For this review, use the dimensioned drawing (mm, ordinates from the lowest corner) and the shaded views. Coordinates: 2 decimals unless noted, no trailing zeros. Order: outer loops, then holes, each group sorted by start corner. A loop starts at its lowest first (then second) coordinate and runs counter-clockwise, first axis right, second up. Notation, with made-up numbers: M -5,-30.75 L 49,-30.75 A10 ccw 49,-14.75 Z; hole C -12.75,63.25 d5. An arc over 180 degrees is marked long. Answer as CSV lines item,"result". Start each with the question number.
Q1. Wall thickness on L1, parallel to Y at x = 6.25, z = 7.75; L2, parallel to Z at x = 3.75, y = 1.25; L3, parallel to Z at x = 8.25, y = 6.5: over which ranges is each line inside the solid? List them lowest first. Write a range as [from, to].
Q2. The part is to be moulded in two halves that separate along X. For the marked faces 1, 2 and 3, say which applies: +X half, -X half, draft (parallel to the pull), parting line (faces both ways), or undercut.
Q3. Consider section D-D on y = 9.75. Write out the cut boundary in (x, z).
Q4. Consider section C-C on x = 8.8. Write out the cut boundary in (y, z).
Q5. For P1, Ø1.2, axis at x = 8.5, z = 6, coming from the -Y side; P2, Ø3, axis at x = 3.5, y = 7, coming from the +Z side; P3, Ø3, axis at x = 6.5, y = 1.5, coming from the +Z side; P4, Ø3, axis at y = 4.5, z = 3.5, coming from the -X side, all flat-tipped, find the tip position at first contact; note any pin that passes through.
Q6. Consider section A-A on z = 6.3. Write out the cut boundary in (x, y).
Q7. Consider section B-B on y = 2. Write out the cut boundary in (x, z), and give its area (3 significant figures).
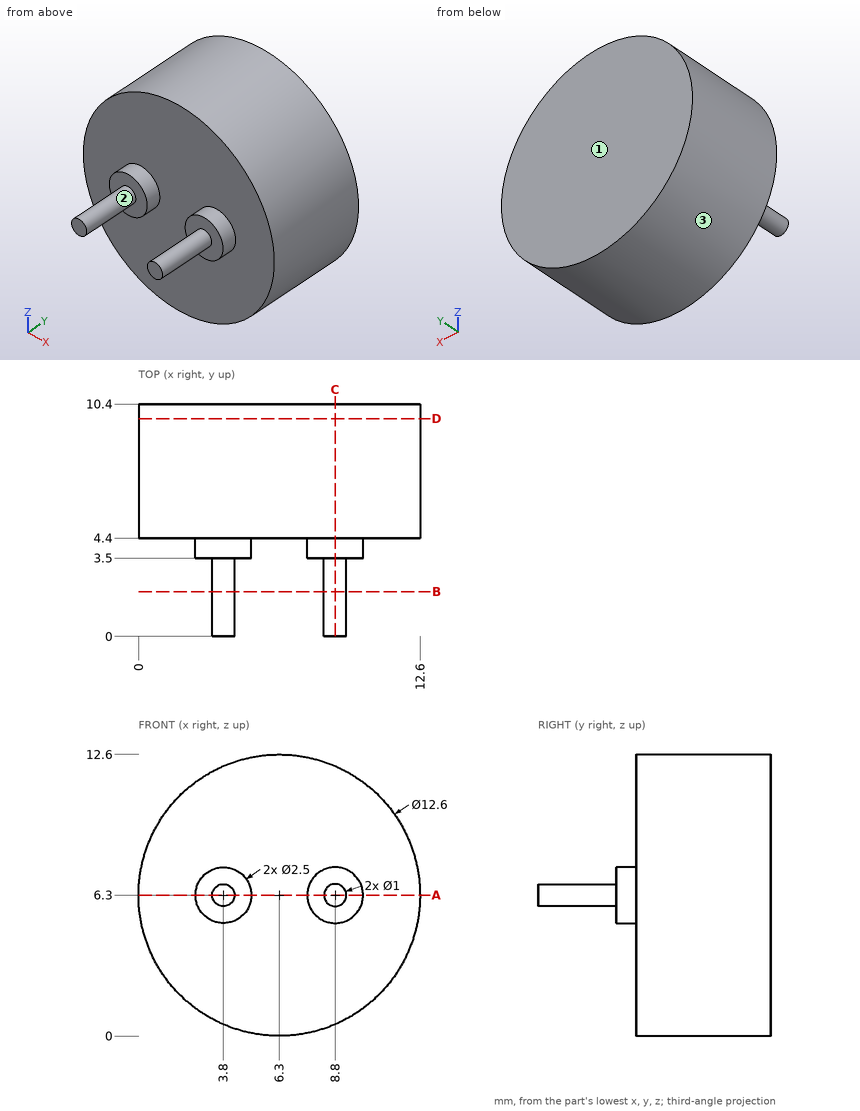
Evaluation:
1,L1,"y = [4.4, 10.4]"
1,L2,"z = [5.8, 6.8]"
1,L3,"z = [0.31, 12.29]"
2,face 1,"draft"
2,face 2,"undercut"
2,face 3,"parting line"
3,outline,"C 6.3,6.3 d12.6"
4,outline,"M 0,5.8 L 3.5,5.8 L 3.5,5.05 L 4.4,5.05 L 4.4,0.52 L 10.4,0.52 L 10.4,12.08 L 4.4,12.08 L 4.4,7.55 L 3.5,7.55 L 3.5,6.8 L 0,6.8 Z"
5,P1,"stops at y = 0"
5,P2,"stops at z = 12.46"
5,P3,"passes through"
5,P4,"stops at x = 0.14"
6,outline,"M 0,4.4 L 2.55,4.4 L 2.55,3.5 L 3.3,3.5 L 3.3,0 L 4.3,0 L 4.3,3.5 L 5.05,3.5 L 5.05,4.4 L 7.55,4.4 L 7.55,3.5 L 8.3,3.5 L 8.3,0 L 9.3,0 L 9.3,3.5 L 10.05,3.5 L 10.05,4.4 L 12.6,4.4 L 12.6,10.4 L 0,10.4 Z"
7,outline,"C 3.8,6.3 d1; C 8.8,6.3 d1"
7,area,"1.57 mm²"
